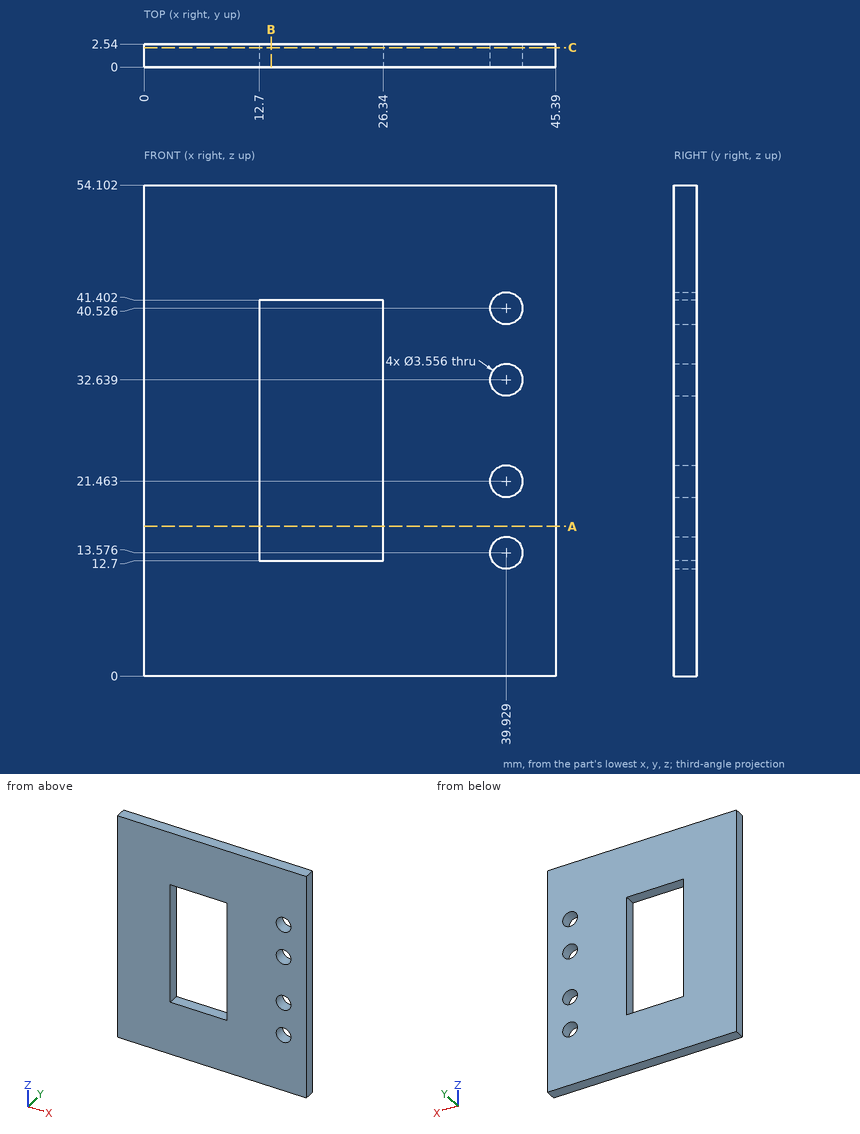
Job drawing, mm, ordinate dimensions from the low corner. One solid piece. Give positions to 0.01 mm unless a question says otherwise; leave off trailing zeros. Loops run counter-clockwise (first coordinate to the right, second up) from the corner with the lowest first, then second, coordinate; pieces in that order, holes last. Notation, with made-up numbers: M 17.25,-5.75 L 46.25,-5.75 A17 cw 46.25,19.25 Z; hole C 36,-1 d7. An arc over 180 degrees is marked long. Answer in a Markdown table with one row per item. Add a question column.
Item 1: Band-saw the part on B-B on x = 14. Give the cut face in (y, z).
Item 2: Band-saw the part on C-C on y = 2.15. Give the cut face in (x, z).
Item 3: Probe probe 1 along Z at (x, y) = (40, 2.25) (1 decimal); probe 2 along X at (y, z) = (2.1, 28); probe 3 along Z at (x, y) = (14, 2.4). List the from-to ranges inside material, lowest first.
Item 4: Band-saw the part on A-A on z = 16.5. Give the cut face in (x, y).
Reply:
| question | item | result |
|---|---|---|
| 1 | outline | M 0,0 L 2.54,0 L 2.54,12.7 L 0,12.7 Z; M 0,41.4 L 2.54,41.4 L 2.54,54.1 L 0,54.1 Z |
| 2 | outline | M 0,0 L 45.39,0 L 45.39,54.1 L 0,54.1 Z; hole M 12.7,12.7 L 26.34,12.7 L 26.34,41.4 L 12.7,41.4 Z; hole C 39.93,13.58 d3.56; hole C 39.93,21.46 d3.56; hole C 39.93,32.64 d3.56; hole C 39.93,40.53 d3.56 |
| 3 | probe 1 | z = 0 to 11.8, 15.4 to 19.7, 23.2 to 30.9, 34.4 to 38.7, 42.3 to 54.1 |
| 3 | probe 2 | x = 0 to 12.7, 26.34 to 45.39 |
| 3 | probe 3 | z = 0 to 12.7, 41.4 to 54.1 |
| 4 | outline | M 0,0 L 12.7,0 L 12.7,2.54 L 0,2.54 Z; M 26.34,0 L 45.39,0 L 45.39,2.54 L 26.34,2.54 Z |
